```python
from build123d import *

# Parameters (mm, degrees)
F0_R          = 1.5
F0_W          = 3.5
F0_H          = 16
F1_DEPTH      = 3
F2_R          = 2.25
F3_DEPTH      = 3
F5_DEPTH      = 1
F5_DEPTH_BACK = 1
F7_R          = 2.25
F8_DEPTH      = 3


with BuildPart() as f1:
    # F0 (on Top) → F1 (new body)
    with BuildSketch(Plane.XY):
        with BuildLine():
            Line((3.5, 8), (3.5, -8))
            Line((3.5, -8), (22, -8))
            ThreePointArc((22, -8), (24.12132, -7.12132), (25, -5))
            Line((25, -5), (25, 5))
            ThreePointArc((25, 5), (24.12132, 7.12132), (22, 8))
            Line((22, 8), (3.5, 8))
        make_face()
        with Locations((9, -4)):
            Circle(F0_R, mode=Mode.SUBTRACT)
        with Locations((15, -4)):
            Circle(F0_R, mode=Mode.SUBTRACT)
        with Locations((21, -4)):
            Circle(F0_R, mode=Mode.SUBTRACT)
        with Locations((9, 4)):
            Circle(F0_R, mode=Mode.SUBTRACT)
        with Locations((15, 4)):
            Circle(F0_R, mode=Mode.SUBTRACT)
        with Locations((21, 4)):
            Circle(F0_R, mode=Mode.SUBTRACT)
        with Locations((1.75, 0)):
            Rectangle(F0_W, F0_H)
    extrude(amount=F1_DEPTH)

    # F2 (on Right) → F3 (join)
    with BuildSketch(Plane.YZ):
        with BuildLine():
            Line((8, 2.719934), (4.97062, 30.541236))
            ThreePointArc((4.97062, 30.541236), (0, 35), (-4.97062, 30.541236))
            Line((-4.97062, 30.541236), (-8, 2.719934))
            Line((-8, 2.719934), (8, 2.719934))
        make_face()
        with Locations((0, 30)):
            Circle(F2_R, mode=Mode.SUBTRACT)
    extrude(amount=F3_DEPTH)

    # F4 (on Front) → F5 (join, two sides)
    with BuildSketch(Plane.XZ) as f5_sk:
        Polygon((9, 25), (0, 25), (0, 2.631591), (24.820279, 2.631591), align=None)
    extrude(amount=F5_DEPTH)
    extrude(f5_sk.sketch, amount=-F5_DEPTH_BACK)

    # F7 (on offset) → F8 (join)
    with BuildSketch(Plane.YZ.offset(9.3)):
        with BuildLine():
            ThreePointArc((3.185419, 27.58068), (3.790889, 28.723613), (4, 30))
            ThreePointArc((4, 30), (-1.276387, 33.790889), (-3.185419, 27.58068))
            ThreePointArc((-3.185419, 27.58068), (0, 26), (3.185419, 27.58068))
        make_face()
        with Locations((0, 30)):
            Circle(F7_R, mode=Mode.SUBTRACT)
        with BuildLine():
            ThreePointArc((3.185419, 27.58068), (0, 26), (-3.185419, 27.58068))
            Line((-3.185419, 27.58068), (0, 0))
            Line((0, 0), (3.185419, 27.58068))
        make_face()
    extrude(amount=F8_DEPTH)


solid = f1.part
```
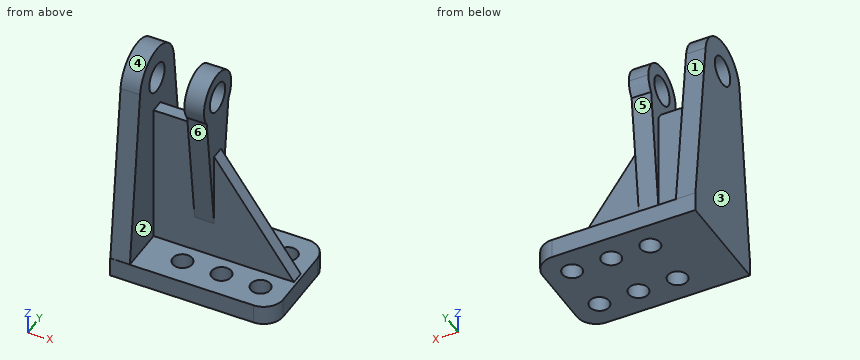
Geometry: final body of the model. Coordinates: model frame, mm. Face numbers are marked on the shaded views. A direction names the side the tool comes from. Give positions to 0.01 mm unless a question says otherwise; leave off trailing zeros. Loops run counter-clockwise (first coordinate to the right, second up) from the corner with the lowest first, then second, coordinate; pieces in that order, holes last. Notation, with made-up numbers: (-35, -33.5) -> (-27, -33.5) arc R24 ccw to (-27, -2.5) -> close; hole circle Ø10 at (-10.75, -18). An arc over 180 degrees is marked (long way). Use one line per item in the form item = value.
Item 1: Access query for the marked faces 4, 5 and 6. Directions: +Z, -Z, +X, -X, +Y, -Y. A direction counts if a zero-diameter tool reaches every point of the face in a straight line with its end or side. Return the directions, or none.
A:
face_4 = +Z, +X, -X
face_5 = +X, +Y
face_6 = +X, -Y
Item 2: Section query B-B on y = 0. Output: boundary loops of the cut face in (x, z).
A:
outline = (0, 0) -> (25, 0) -> (25, 3) -> (24.56, 3) -> (12.3, 20.33) -> (12.3, 27.75) -> (9.3, 27.75) -> (9.3, 24.58) -> (9, 25) -> (3, 25) -> (3, 27.75) -> (0, 27.75) -> close; (0, 32.25) -> (3, 32.25) -> (3, 35) -> (0, 35) -> close; (9.3, 32.25) -> (12.3, 32.25) -> (12.3, 34) -> (9.3, 34) -> close
Item 3: Line query: probe 1 along Y at (x, z) = (21, 2.45); probe 2 along X at (y, z) = (2.75, 31.5); probe 3 along Z at (x, y) = (10.75, 0). Output: solid intervals per line, ascending.
A:
probe_1 = -8 to -5.5, -2.5 to 2.5, 5.5 to 8
probe_2 = 0 to 3, 9.3 to 12.3
probe_3 = 0 to 27.75, 32.25 to 34
Item 4: Section query D-D on x = 21.5. Output: boundary loops of the cut face in (y, z), and give its area (3 significant figures).
A:
outline = (-8, 0) -> (-5.41, 0) -> (-5.41, 3) -> (-8, 3) -> close; (-2.59, 0) -> (2.59, 0) -> (2.59, 3) -> (1, 3) -> (1, 7.33) -> (-1, 7.33) -> (-1, 3) -> (-2.59, 3) -> close; (5.41, 0) -> (8, 0) -> (8, 3) -> (5.41, 3) -> close
area = 39.7 mm^2
Item 5: Section query C-C on x = 5. Output: boundary loops of the cut face in (y, z), and give its area (3 significant figures).
A:
outline = (-8, 0) -> (8, 0) -> (8, 3) -> (1, 3) -> (1, 25) -> (-1, 25) -> (-1, 3) -> (-8, 3) -> close
area = 92.0 mm^2
Item 6: Section query A-A on x = 11.25. Output: boundary loops of the cut face in (y, z).
A:
outline = (-8, 0) -> (8, 0) -> (8, 3) -> (1, 3) -> (1, 8.66) -> (3.19, 27.58) arc R4 ccw to (4, 30) arc R4 ccw (long way) to (-3.19, 27.58) -> (-1, 8.66) -> (-1, 3) -> (-8, 3) -> close; hole circle Ø4.5 at (0, 30)
Item 7: Draft query along X for the marked faces 1, 2 and 3. Return one class per face: pulls with the +X half, pulls with the -X half, needs draft (parallel to the pull), parting line crosses it, or undercut.
A:
face_1 = needs draft
face_2 = undercut
face_3 = pulls with the -X half
Item 8: Pin query (flat end, axial travel): P1, Ø6, axis at x = 7, y = -3, coming from the +Z side; P2, Ø1.5, axis at x = 14, z = 27.5, coming from the +Y side; P3, Ø2, axis at x = 6.5, y = -0.5, coming from the +Z side; P4, Ø3.5, axis at x = 21, y = -4, coming from the +Z side. Return the tip coordinate at first contact, or that it passes through.
A:
P1 = 33.85
P2 = through
P3 = 25
P4 = 3
